```python
from build123d import *

# Parameters (mm, degrees)
ESQUISSE1_R        = 1.5
BOSS_EXTRU_2_DEPTH = 6
CONG_2_R           = 2
CONG_3_R           = 10


with BuildPart() as part:
    # Esquisse1 → Boss.-Extru.2 (new body)
    with BuildSketch(Plane(origin=(0, 0, 0), x_dir=(1, 0, 0), z_dir=(0, 1, 0))):
        with BuildLine():
            Line((0, 0), (17, 0))
            Line((17, 0), (17, 15))
            ThreePointArc((17, 15), (25.571067812, 17.307611845), (30, 25))
            ThreePointArc((30, 25), (25.571067812, 32.692388155), (17, 35))
            Line((17, 35), (17, 50))
            Line((17, 50), (0, 50))
            Line((0, 50), (0, 0))
        make_face()
        with BuildLine():
            ThreePointArc((5.798134367, 22.5), (8.5, 25.201865633), (11.201865633, 22.5))
            Line((11.201865633, 22.5), (11.201865633, 19.857230824))
            ThreePointArc((11.201865633, 19.857230824), (8.5, 8.5), (5.798134367, 19.857230824))
            Line((5.798134367, 19.857230824), (5.798134367, 22.5))
        make_face(mode=Mode.SUBTRACT)
        with Locations(Location((23.5, 25, 0), (0, 0, 270))):
            Circle(ESQUISSE1_R, mode=Mode.SUBTRACT)
    extrude(amount=BOSS_EXTRU_2_DEPTH)

    # Congé2
    cong_2_edges = [part.edges().sort_by_distance(p)[0] for p in [
        (17, 3, 0),
        (0, 3, 0),
        (0, 3, -50),
        (17, 3, -50),
    ]]
    fillet(cong_2_edges, radius=CONG_2_R)

    # Congé3
    # the kernel refuses this fillet: 10 mm, written as the material it takes off along each edge
    with BuildSketch(Plane(origin=(30, -30.063050545, -25), x_dir=(-0.6246887700874293, 0, 0.7808738313752451), z_dir=(0, 1, 0))) as cong_3_piece_1:
        with BuildLine():
            CenterArc((6.840779647, -8.551115481), CONG_3_R, 58.772060321, 139.774574658)
            ThreePointArc((-2.639871114, -11.731879721), (-2.959277225, -5.497060293), (0, 0))
            ThreePointArc((0, 0), (6.012610109, 1.680331289), (12.025220218, 0))
        make_face()
    extrude(amount=66.126101089, mode=Mode.SUBTRACT)


solid = part.part
```
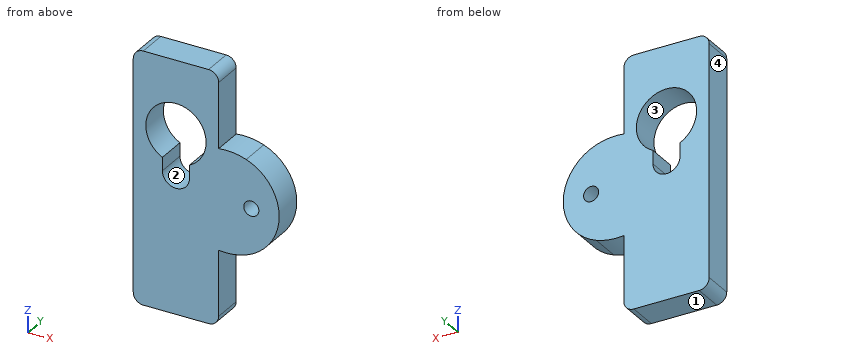
The model under review builds one solid part; all positions refer to its coordinate system, in mm. Face numbers are marked on the shaded views. Coordinates: 2 decimals unless noted, no trailing zeros. Order: outer loops, then holes, each group sorted by start corner. A loop starts at its lowest first (then second) coordinate and runs counter-clockwise, first axis right, second up. Notation, with made-up numbers: (59, -32.75) -> (82, -32.75) arc R25 cw to (82, 6.25) -> close; hole circle Ø1 at (54, -27.5). An arc over 180 degrees is marked (long way). Answer in a Markdown table with one row per item. Add a question column.
Item 1: We need section D-D on z = -44.5. Write out the cut boundary in (x, y).
Item 2: We need section A-A on x = 8.5. Write out the cut boundary in (y, z).
Item 3: We need section B-B on y = 1.6. Write out the cut boundary in (x, z), plus the area to 3 significant figures.
Item 4: Mouldability with a two-part tool opening along Z and no side actions: class the marked faces 1, 2, 3 and 4 as +Z half, -Z half, draft (parallel to the pull), parting line (faces both ways), or undercut.
Item 5: Clearance check with flat-ended pins moving along their axes: pin 1 (3 mm diameter, centred on y = 2, z = -43.5, fed in from +X); pin 2 (1.3 mm diameter, centred on y = 3.5, z = -22, fed in from +X). State where each tip first meets the part, or that it passes through.
Item 6: To check wall thickness, follow probe 1 along X at (y, z) = (1.5, -14.5); probe 2 along Z at (x, y) = (8.5, 3.15); probe 3 along Z at (x, y) = (12, 4.5). State the ranges of each line that lie inside material, in increasing order.
Item 7: We need section C-C on z = -17.5. Write out the cut boundary in (x, y).
Final values:
| question | item | result |
|---|---|---|
| 1 | outline | (0, 0) -> (17, 0) -> (17, 6) -> (0, 6) -> close |
| 2 | outline | (0, -50) -> (6, -50) -> (6, -25.2) -> (0, -25.2) -> close; (0, -8.5) -> (6, -8.5) -> (6, 0) -> (0, 0) -> close |
| 3 | outline | (0, -48) arc R2 ccw to (2, -50) -> (15, -50) arc R2 ccw to (17, -48) -> (17, -35) arc R11.6 ccw to (22.49, -34.39) arc R10 ccw to (22.49, -15.61) arc R11.6 ccw to (17, -15) -> (17, -2) arc R2 ccw to (15, 0) -> (2, 0) arc R2 ccw to (0, -2) -> close; hole (5.8, -22.5) arc R2.7 ccw to (11.2, -22.5) -> (11.2, -19.86) arc R6 ccw (long way) to (5.8, -19.86) -> close; hole circle Ø3 at (23.5, -25) |
| 3 | area | 902 mm2 |
| 4 | face 1 | -Z half |
| 4 | face 2 | undercut |
| 4 | face 3 | undercut |
| 4 | face 4 | draft |
| 5 | pin 1 | stops at x = 17 |
| 5 | pin 2 | stops at x = 28.77 |
| 6 | probe 1 | x = 0 to 2.5, 14.5 to 17 |
| 6 | probe 2 | z = -50 to -25.2, -8.5 to 0 |
| 6 | probe 3 | z = -50 to -19.37, -9.63 to 0 |
| 7 | outline | (0, 0) -> (3.3, 0) -> (3.3, 6) -> (0, 6) -> close; (13.7, 0) -> (25.66, 0) -> (25.66, 6) -> (13.7, 6) -> close |
